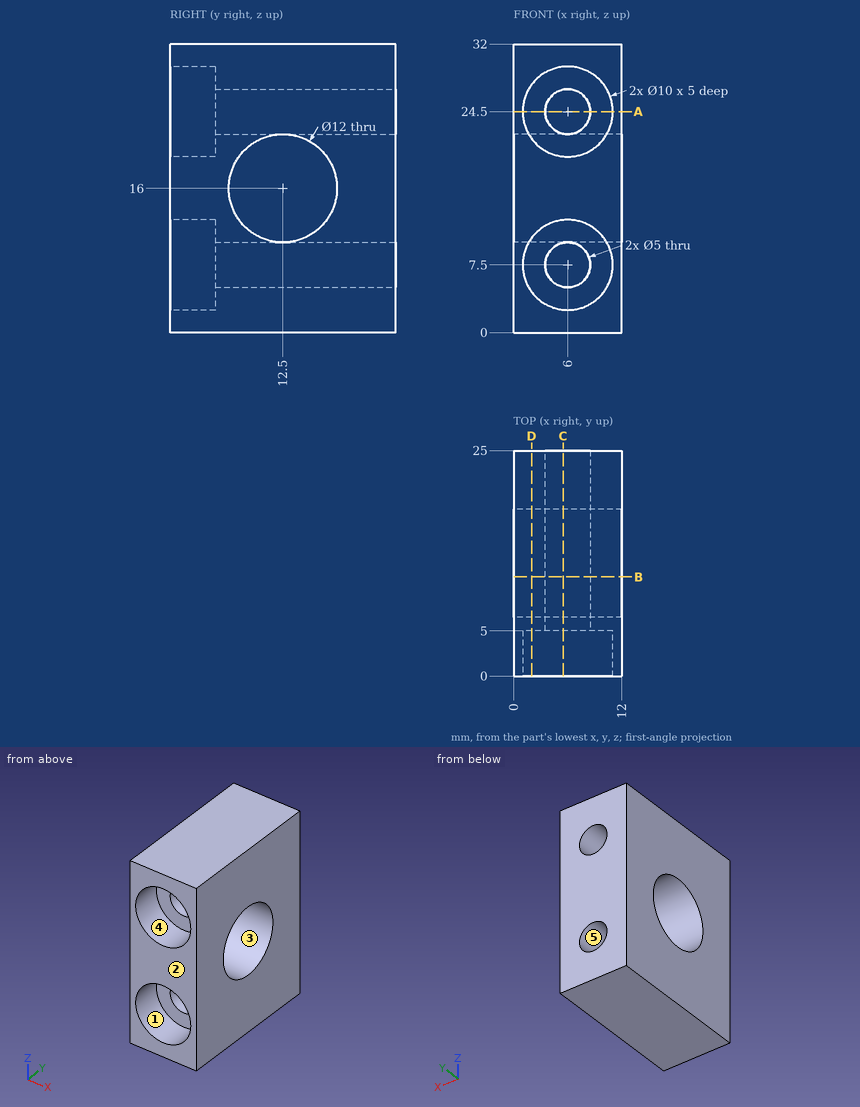
Here's the drawing with two shaded views (mm, measured from the low corner). I have some questions. A direction names the side the tool comes from. Give positions to 0.01 mm unless a question says otherwise; leave off trailing zeros. Write each loop counter-clockwise with the first axis right and the second up, starting at its lowest first coordinate (ties: lowest second). Pieces come first, ordered by that corner, then holes. Notation, with made-up numbers: (29, 0.25) -> (63, 0.25) arc R18 ccw to (63, 33.25) -> close; hole circle Ø9 at (-13.5, -15.75). An arc over 180 degrees is marked (long way). Use one line per item in the form item = value.
1) On a 3-axis mill with a long thin cutter (end or side, diameter ignored), from which of +Z, -Z, +X, -X, +Y, -Y can I reach the whole of each face in a straight line? I mean the marked faces 4 and 5. Say none if no direction works.
Verdict:
face_4 = -Y
face_5 = +Y, -Y
2) Suppose I cut it at D-D (x = 2). Please give me the cut outline in (y, z).
Verdict:
outline = (0, 0) -> (25, 0) -> (25, 32) -> (0, 32) -> (0, 27.5) -> (5, 27.5) -> (5, 21.5) -> (0, 21.5) -> (0, 10.5) -> (5, 10.5) -> (5, 4.5) -> (0, 4.5) -> close; hole circle Ø12 at (12.5, 16)
3) I'm going to push flat-ended pins straight in: pin 1 (4.5 mm diameter, centred on x = 6, z = 24.5, fed in from +Y); pin 2 (5 mm diameter, centred on x = 7, z = 5.5, fed in from -Y). Where does each tip first touch, or does it pass through?
Verdict:
pin_1 = through
pin_2 = 5
4) If I drill on L1, parallel to Z at x = 6, y = 4.05; L2, parallel to Y at x = 8.25, z = 16; L3, parallel to Z at x = 8.75, y = 12.5, over which ranges is the centre line in solid material (lowest first)? Write a range as [from, to].
Verdict:
L1 = [0, 2.5], [12.5, 19.5], [29.5, 32]
L2 = [0, 6.5], [18.5, 25]
L3 = [0, 10], [22, 32]
5) Suppose I cut it at C-C (x = 5.5). Please give me the cut outline in (y, z).
Verdict:
outline = (0, 0) -> (25, 0) -> (25, 5.05) -> (5, 5.05) -> (5, 2.53) -> (0, 2.53) -> close; (0, 12.47) -> (5, 12.47) -> (5, 9.95) -> (25, 9.95) -> (25, 22.05) -> (5, 22.05) -> (5, 19.53) -> (0, 19.53) -> close; (0, 29.47) -> (5, 29.47) -> (5, 26.95) -> (25, 26.95) -> (25, 32) -> (0, 32) -> close; hole circle Ø12 at (12.5, 16)
6) Suppose I cut it at A-A (z = 24.5). Please give me the cut outline in (x, y).
Verdict:
outline = (0, 0) -> (1, 0) -> (1, 5) -> (3.5, 5) -> (3.5, 25) -> (0, 25) -> close; (8.5, 5) -> (11, 5) -> (11, 0) -> (12, 0) -> (12, 25) -> (8.5, 25) -> close
7) Suppose I cut it at B-B (y = 11). Please give me the cut outline in (x, z), and give its area (3 significant figures).
Verdict:
outline = (0, 0) -> (12, 0) -> (12, 10.19) -> (0, 10.19) -> close; (0, 21.81) -> (12, 21.81) -> (12, 32) -> (0, 32) -> close; hole circle Ø5 at (6, 7.5); hole circle Ø5 at (6, 24.5)
area = 205 mm2
8) We'd pull the mould along Y, two halves only. Please class the marked faces 1, 2 and 3: +Y half, -Y half, draft (parallel to the pull), parting line (faces both ways), or undercut.
Verdict:
face_1 = draft
face_2 = -Y half
face_3 = undercut
